Part print with two shaded views. Sizes in mm from the minimum x, y, z corner. A direction names the side the tool comes from. Round coordinates to 2 decimals unless told otherwise and drop trailing zeros. Loops run counter-clockwise (first coordinate to the right, second up) from the corner with the lowest first, then second, coordinate; pieces in that order, holes last. Notation, with made-up numbers: M -36.5,73 L -20.5,73 A26 cw -20.5,111 Z; hole C 66.25,49.5 d11. An arc over 180 degrees is marked long. Use a Markdown table: item, result. Add a question column.
Item 1: Saw through at D-D on x = 12.5. Write the cut outline in (y, z), then the cut area to 3 significant figures.
Item 2: Pin check, flat tips, straight feed: P1, Ø6, axis at x = 3, y = 36, coming from the -Z side; P2, Ø4, axis at x = 15.5, y = 22, coming from the +Z side; P3, Ø10, axis at y = 46, z = 20, coming from the +X side. Stop position of each tip, or through.
Item 3: Saw through at A-A on z = 12.5. Write the cut outline in (x, y).
Item 4: Wall check: L1, parallel to Y at x = 12.5, z = 4.5; L2, parallel to Y at x = 10, z = 11; L3, parallel to Z at x = 1.75, y = 12.5. Give the ranges that are in metal, low to high. Write a range as from..to.
Item 5: Saw through at C-C on y = 45.5. Write the cut outline in (x, z).
Item 6: Saw through at B-B on x = 17. Write the cut outline in (y, z).
Item 7: Tool access for the marked faces 1, 2 and 3: list every direction of +Z, -Z, +X, -X, +Y, -Y with a clear straight run to the whole face (end or side of a thin tool).
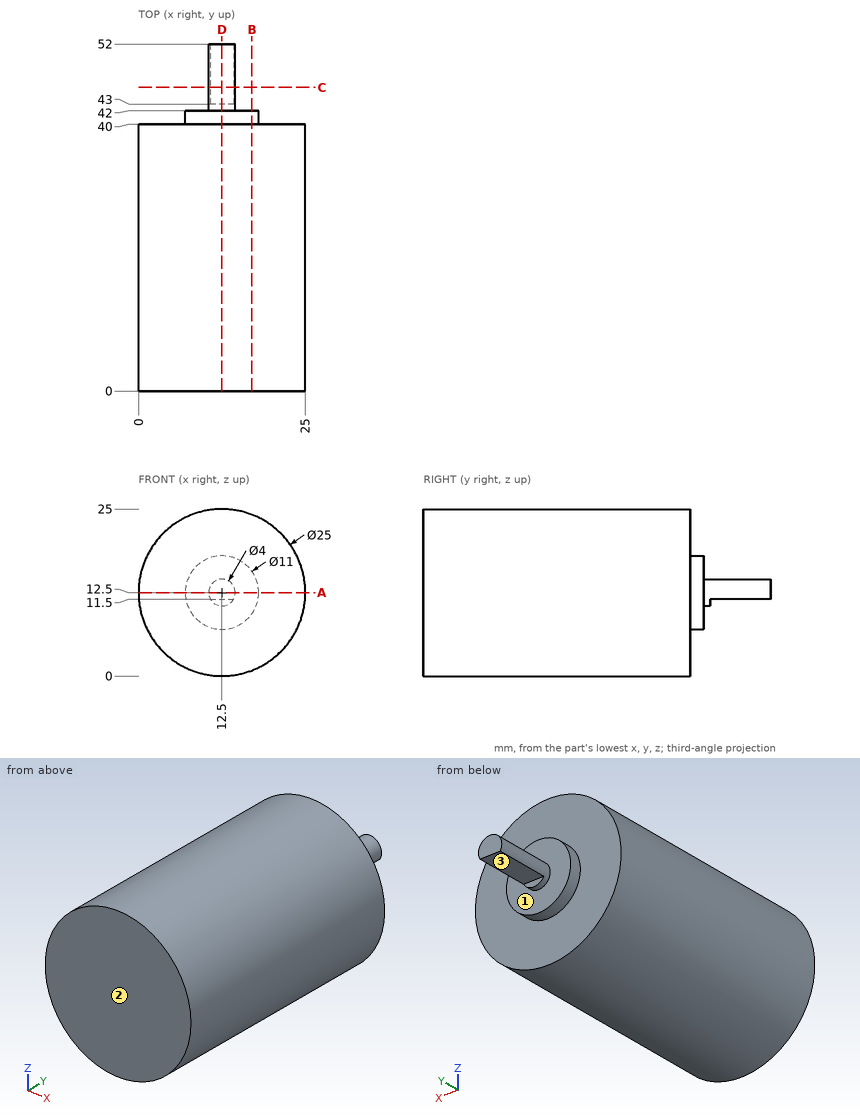
Entries:
| question | item | result |
|---|---|---|
| 1 | outline | M 0,0 L 40,0 L 40,7 L 42,7 L 42,10.5 L 43,10.5 L 43,11.5 L 52,11.5 L 52,14.5 L 42,14.5 L 42,18 L 40,18 L 40,25 L 0,25 Z |
| 1 | area | 1,050 mm2 |
| 2 | P1 | z = 1.82 |
| 2 | P2 | z = 24.96 |
| 2 | P3 | x = 15.66 |
| 3 | outline | M 0,0 L 25,0 L 25,40 L 18,40 L 18,42 L 14.5,42 L 14.5,52 L 10.5,52 L 10.5,42 L 7,42 L 7,40 L 0,40 Z |
| 4 | L1 | 0..40 |
| 4 | L2 | 0..42 |
| 4 | L3 | 6.12..18.88 |
| 5 | outline | M 10.77,11.5 L 14.23,11.5 A2 ccw long Z |
| 6 | outline | M 0,0.84 L 40,0.84 L 40,9.34 L 42,9.34 L 42,15.66 L 40,15.66 L 40,24.16 L 0,24.16 Z |
| 7 | face 1 | +Y |
| 7 | face 2 | +Z, -Z, +X, -X, -Y |
| 7 | face 3 | -Z, +X, -X, +Y |
